from build123d import *

# Parameters (mm, degrees)
CROQUIS1_W              = 180
CROQUIS1_H              = 180
SALIENTE_EXTRUIR1_DEPTH = 30.7
CROQUIS2_W              = 162.99
CROQUIS2_H              = 162.21
CORTAR_EXTRUIR1_DEPTH   = 20.7
CROQUIS4_W              = 175
CROQUIS4_H              = 10.7
CORTAR_EXTRUIR2_DEPTH   = 175
CORTAR_EXTRUIR3_REACH   = 258.403
CROQUIS5_W              = 30.7
CROQUIS5_H              = 38
CROQUIS6_W              = 82.99
CROQUIS6_H              = 38
CORTAR_EXTRUIR4_DEPTH   = 5
CROQUIS7_W              = 6.8
CROQUIS7_H              = 70
CORTAR_EXTRUIR5_DEPTH   = 5
CROQUIS8_W              = 175
CROQUIS8_H              = 50
CORTAR_EXTRUIR6_DEPTH   = 3
CHAFL_N1_SIZE           = 15
CHAFL_N1_SIZE2          = 8.660254038
CROQUIS9_R              = 1.4
CORTAR_EXTRUIR7_DEPTH   = 20


with BuildPart() as part:
    # Croquis1 → Saliente-Extruir1 (new body)
    with BuildSketch(Plane.XY):
        with Locations((90, 90)):
            Rectangle(CROQUIS1_W, CROQUIS1_H)
    extrude(amount=SALIENTE_EXTRUIR1_DEPTH)

    # Croquis2 → Cortar-Extruir1 (cut)
    with BuildSketch(Plane(origin=(0, 0, 0), x_dir=(-1, 0, 0), z_dir=(0, 0, -1))):
        with Locations((-98.505, 98.895)):
            Rectangle(CROQUIS2_W, CROQUIS2_H)
    extrude(amount=-CORTAR_EXTRUIR1_DEPTH, mode=Mode.SUBTRACT)

    # Croquis4 → Cortar-Extruir2 (cut)
    with BuildSketch(Plane(origin=(0, 180, 0), x_dir=(1, 0, 0), z_dir=(0, 1, 0))):
        with Locations((92.5, -15.35)):
            Rectangle(CROQUIS4_W, CROQUIS4_H)
    extrude(amount=-CORTAR_EXTRUIR2_DEPTH, mode=Mode.SUBTRACT)

    # Cortar-Extruir3: up to this face of the body (flat: up to its plane)
    cortar_extruir3_end = Plane(part.part.faces().sort_by_distance((17.01, 98.895, 5))[0])
    # Croquis5 → Cortar-Extruir3 (cut, up to the picked face)
    with BuildSketch(Plane.ZY, mode=Mode.PRIVATE) as cortar_extruir3_sk1:
        with Locations((15.35, 161)):
            Rectangle(CROQUIS5_W, CROQUIS5_H)
    cortar_extruir3_tool1 = split(extrude(cortar_extruir3_sk1.sketch, amount=-CORTAR_EXTRUIR3_REACH, mode=Mode.PRIVATE), bisect_by=cortar_extruir3_end, keep=Keep.BOTH, mode=Mode.PRIVATE)
    add(cortar_extruir3_tool1.solids().sort_by(Axis((0, 161, 15.35), (1, 0, 0)))[0], mode=Mode.SUBTRACT)

    # Croquis6 → Cortar-Extruir4 (cut)
    with BuildSketch(Plane(origin=(0, 0, 20.7), x_dir=(-1, 0, 0), z_dir=(0, 0, -1))):
        with Locations((-98.505, 161)):
            Rectangle(CROQUIS6_W, CROQUIS6_H)
    extrude(amount=-CORTAR_EXTRUIR4_DEPTH, mode=Mode.SUBTRACT)

    # Croquis7 → Cortar-Extruir5 (cut)
    with BuildSketch(Plane.XY.offset(30.7)):
        with Locations((176.6, 80)):
            Rectangle(CROQUIS7_W, CROQUIS7_H)
    extrude(amount=-CORTAR_EXTRUIR5_DEPTH, mode=Mode.SUBTRACT)

    # Croquis8 → Cortar-Extruir6 (cut)
    with BuildSketch(Plane(origin=(0, 0, 20.7), x_dir=(-1, 0, 0), z_dir=(0, 0, -1))):
        with Locations((-92.5, 30)):
            Rectangle(CROQUIS8_W, CROQUIS8_H)
    extrude(amount=-CORTAR_EXTRUIR6_DEPTH, mode=Mode.SUBTRACT)

    # Chaflán1
    chafl_n1_edges = [part.edges().sort_by_distance(p)[0] for p in [
        (98.505, 17.79, 0),
        (17.01, 79.895, 0),
    ]]
    chafl_n1_side = [part.faces().sort_by_distance(p)[0] for p in [
        (8.505, 139.707315983, 0),
    ]]
    chamfer(chafl_n1_edges, length=CHAFL_N1_SIZE, length2=CHAFL_N1_SIZE2, reference=chafl_n1_side[0])

    # Croquis9 → Cortar-Extruir7 (cut)
    with BuildSketch(Plane.XY.offset(30.7)):
        with Locations((176.6, 65)):
            Circle(CROQUIS9_R)
        with Locations((176.6, 95)):
            Circle(CROQUIS9_R)
        with Locations((120, 161)):
            Circle(CROQUIS9_R)
        with Locations((77.01, 161)):
            Circle(CROQUIS9_R)
    extrude(amount=-CORTAR_EXTRUIR7_DEPTH, mode=Mode.SUBTRACT)


solid = part.part
Build history of the part. All positions in model axes, mm. A direction names the side the tool comes from. Round coordinates to 2 decimals unless told otherwise and drop trailing zeros. Write each loop counter-clockwise with the first axis right and the second up, starting at its lowest first coordinate (ties: lowest second). Pieces come first, ordered by that corner, then holes. Notation, with made-up numbers: (-30, 11.5) - (-1, 11.5) arc R14 cw to (-1, 21.5) - close; hole circle Ø1 at (-36.75, 1.5). An arc over 180 degrees is marked (long way). Use CSV: the item, a comma, the result in double quotes.
(1) Band-saw the part on A-A (x = 108.5). Write the cut outline in (y, z), plus the area to 3 significant figures.
Response:
outline,"(0, 0) - (2.79, 0) - (17.79, 8.66) - (17.79, 10) - (5, 10) - (5, 23.7) - (55, 23.7) - (55, 20.7) - (142, 20.7) - (142, 25.7) - (180, 25.7) - (180, 30.7) - (0, 30.7) - close"
area,"1,630 mm²"
(2) Pin check, flat tips, straight feed: P1, Ø1.5, axis at y = 106, z = 3.5, coming from the +X side; P2, Ø10, axis at x = 95.5, y = 18, coming from the -Z side; P3, Ø2, axis at x = 176.6, y = 95, coming from the -Z side; P4, Ø8, axis at x = 160.5, y = 30, coming from the -Z side. Stop position of each tip, or through.
Response:
P1,"x = 9.37"
P2,"z = 5.89"
P3,"through"
P4,"z = 23.7"
(3) 3-axis set-ups, long thin cutter, end or side, ignore diameter. For faces 4 (the flat face through (9.61, 71.42, 4.39)), 5 (the flat face through (4.6, 142, 18.5)), 6 (the flat face through (177, 45, 28)): which of +Z, -Z, +X, -X, +Y, -Y reach the whole face in a straight line?
Response:
face 4,"-Z, +X, +Y"
face 5,"+Z, -Z, -X, +Y"
face 6,"+Z, +X"
(4) Mould opens along Z. For faces 1 (the flat face through (99, 142, 23)), 2 (the flat face through (91, 5, 17)), 3 (the flat face through (177, 80, 25.7)) say: pulls with the +Z half, pulls with the -Z half, needs draft (parallel to the pull), parting line crosses it, or undercut.
Response:
face 1,"needs draft"
face 2,"undercut"
face 3,"pulls with the +Z half"
(5) Wall check: line 1 (X direction, y = 161, z = 28); line 2 (X direction, y = 95, z = 24); line 3 (Y direction, x = 84.5, z = 17). Give the ranges that are in metal, low to high.
Response:
line 1,"17.01 to 75.61, 78.41 to 118.6, 121.4 to 180"
line 2,"0 to 175.2, 178 to 180"
line 3,"0 to 5"
(6) Band-saw the part on B-B (z = 15.5). Write the cut outline in (x, y).
Response:
outline,"(0, 0) - (180, 0) - (180, 5) - (5, 5) - (5, 142) - (0, 142) - close"
(7) Band-saw the part on C-C (y = 40.5). Write the cut outline in (x, z).
Response:
outline,"(0, 0) - (2.01, 0) - (17.01, 8.66) - (17.01, 10) - (5, 10) - (5, 23.7) - (180, 23.7) - (180, 30.7) - (0, 30.7) - close"
